Solid Edge part; units mm, degrees
sketch "Sketch1" plane through (0, 0, 0) normal (0, 0, 1) x (1, 0, 0)
  arc A0 (28.356, 57.3753) -> (61.1888, -18.76) centre (0, -0.0001) cw
  line L0 (57.1313, -28.8447) -> (61.1888, -18.76)
  arc A1 (57.1313, -28.8447) -> (28.8478, -57.1298) centre (0, -0.0001) cw
  line L1 (18.7636, -61.1877) -> (28.8478, -57.1298)
  arc A2 (18.7636, -61.1877) -> (5.0002, -63.8044) centre (0, -0.0001) cw
  line L2 (5.0002, -63.8044) -> (5.0002, -62.2996)
  line L3 (6.0906, 63.7095) -> (6.0906, 62.2025)
  arc A3 (6.0906, 63.7095) -> (19.0724, 61.092) centre (0, -0.0001) cw
  line L4 (19.0724, 61.092) -> (28.356, 57.3753)
  arc A4 (6.0906, 62.2025) -> (5.0002, -62.2997) centre (0, 0) cw
  arc A5 (6.0906, 62.2025) -> (5.0002, -62.2997) centre (0, 0) cw
  arc A6 (6.0906, 62.2025) -> (5.0002, -62.2997) centre (0, 0) cw
extrude "Protrusion1" add sketch "Sketch1" against normal blind 30
hole "Hole_3" at (23.7398, -59.1853, -5.9053) direction (-0.3733, 0.9277, 0) diameter 2.5 end up to next
hole "Hole1" at (23.8716, -59.1322, -24.3079) direction (-0.3733, 0.9277, 0) diameter 2.5 end up to next
hole "Hole2" at (23.7398, -59.1853, -15) direction (-0.3733, 0.9277, 0) diameter 2.5 end up to next
hole "Hole_6" at (23.7194, 59.2316, -3.97) direction (-0.3717, -0.9284, 0) diameter 2.5 end up to next
hole "Hole3" at (23.6662, 59.2529, -15.0704) direction (-0.3717, -0.9284, 0) diameter 2.5 end up to next
hole "Hole4" at (23.6447, 59.2615, -24.9501) direction (-0.3717, -0.9284, 0) diameter 2.5 end up to next
The listing builds one solid part. Answer for the finished solid, in the listing's coordinates (mm). Coordinates: 2 decimals unless noted, no trailing zeros. Loops run counter-clockwise (first coordinate to the right, second up) from the corner with the lowest first, then second, coordinate; pieces in that order, holes last. Notation, with made-up numbers: (83, -14.75) - (123, -14.75) arc R18 cw to (123, 6.25) - close; hole circle Ø11 at (65.25, -14). An arc over 180 degrees is marked (long way). Use a Markdown table: item, result. Add a question column.
1) Find the intervals of material crossed by line 1 (Y direction, x = 20, z = -18); line 2 (Y direction, x = 40.5, z = -3); line 3 (X direction, y = -15.5, z = -27), in increasing order.
2) The part is cut by section B-B, the plane z = -11.5. Give the vertices of the cut face in (x, y), and give its area (3 significant figures).
3) The part is cut by section C-C, the plane x = 11. Give the vertices of the cut face in (y, z), and give its area (3 significant figures).
4) The part is cut by section D-D, the plane y = -11.5. Give the vertices of the cut face in (x, z).
5) Given pin 1 (1.5 mm diameter, centred on x = 32, z = -3.5, fed in from +Y); pin 2 (2 mm diameter, centred on x = 14.5, z = -19.5, fed in from +Y); pin 3 (3 mm diameter, centred on x = 25, z = -18.5, fed in from -Y), each flat-ended and moving along its own axis, determine where each tip first touches the part or whether it passes through.
6) The part is cut by section A-A, the plane x = 59. Give the vertices of the cut face in (y, z), and give its area (3 significant figures).
7) The mould has two halves that part along X. Classify faces 1 (the flat face through (63, 10, -30)), 2 (the cylindrical face through (23.034, 58.807, -2.815)), 3 (the flat face through (59.132, -23.873, -14.79)), 4 (the cylindrical face through (23.28, -58.67, -25.5)): released by +X, released by -X, zero draft, split by the parting line, or undercut.
Here are the results:
| question | item | result |
|---|---|---|
| 1 | line 1 | y = -60.69 to -59.21, 59.21 to 60.72 |
| 1 | line 2 | y = -49.56 to -47.6, 47.6 to 49.56 |
| 1 | line 3 | x = 60.55 to 62.09 |
| 2 | outline | (5, -63.8) arc R64 ccw to (18.76, -61.19) - (28.85, -57.13) arc R64 ccw to (57.13, -28.84) - (61.19, -18.76) arc R64 ccw to (28.36, 57.38) - (19.07, 61.09) arc R64 ccw to (6.09, 63.71) - (6.09, 62.2) arc R62.5 cw to (5, -62.3) - close |
| 2 | area | 277 mm^2 |
| 3 | outline | (-63.05, -30) - (-61.52, -30) - (-61.52, 0) - (-63.05, 0) - close; (61.52, -30) - (63.05, -30) - (63.05, 0) - (61.52, 0) - close |
| 3 | area | 91.4 mm^2 |
| 4 | outline | (61.43, -30) - (62.96, -30) - (62.96, 0) - (61.43, 0) - close |
| 5 | pin 1 | stops at y = 55.85 |
| 5 | pin 2 | stops at y = 62.56 |
| 5 | pin 3 | stops at y = -59.28 |
| 6 | outline | (-24.2, -30) - (-20.62, -30) - (-20.62, 0) - (-24.2, 0) - close; (20.62, -30) - (24.8, -30) - (24.8, 0) - (20.62, 0) - close |
| 6 | area | 233 mm^2 |
| 7 | face 1 | zero draft |
| 7 | face 2 | undercut |
| 7 | face 3 | released by +X |
| 7 | face 4 | undercut |
